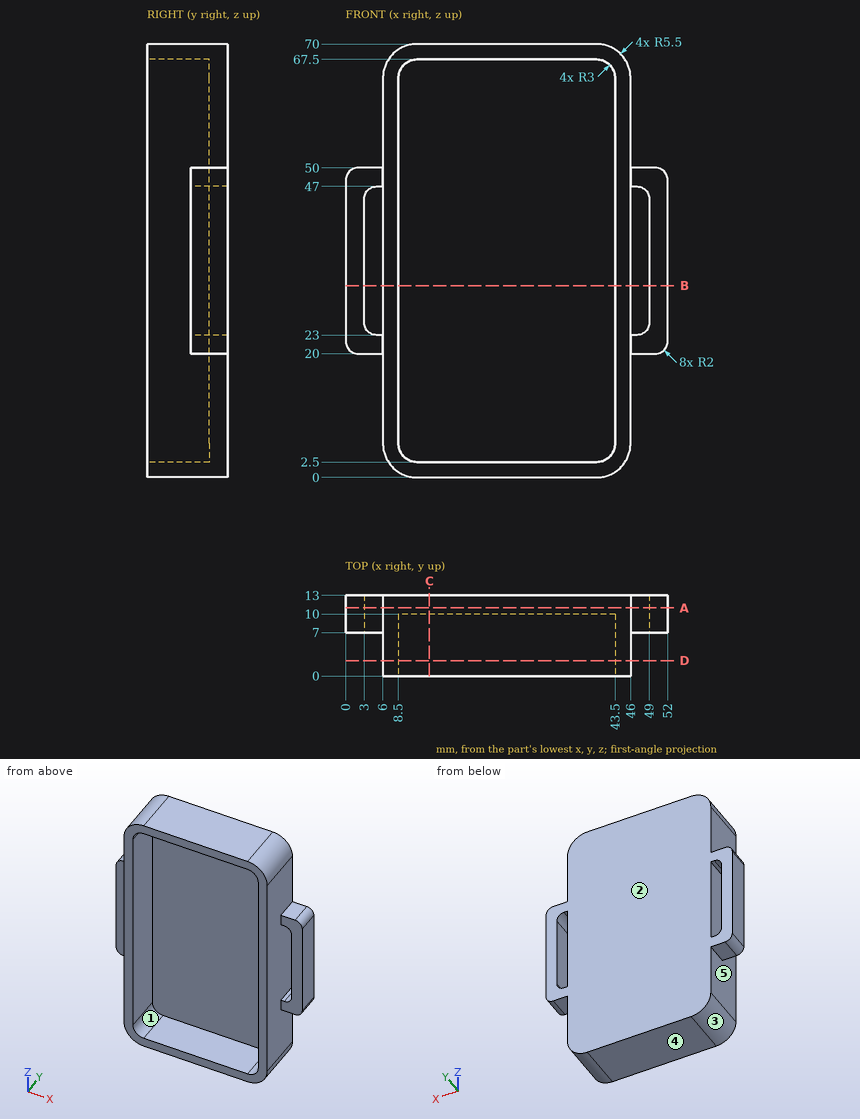
Geometry check sheet. Reference: drawing and pictorial views, mm from the part's lowest x, y, z. A direction names the side the tool comes from. Coordinates: 2 decimals unless noted, no trailing zeros. Order: outer loops, then holes, each group sorted by start corner. A loop starts at its lowest first (then second) coordinate and runs counter-clockwise, first axis right, second up.
1. Sectioned sample at D-D, the plane y = 2.5. Record the cut outline in (x, z), and give its area (3 significant figures).
Results found:
outline: (6, 5.5) arc R5.5 ccw to (11.5, 0) - (40.5, 0) arc R5.5 ccw to (46, 5.5) - (46, 64.5) arc R5.5 ccw to (40.5, 70) - (11.5, 70) arc R5.5 ccw to (6, 64.5) - close; hole (8.5, 5.5) arc R3 ccw to (11.5, 2.5) - (40.5, 2.5) arc R3 ccw to (43.5, 5.5) - (43.5, 64.5) arc R3 ccw to (40.5, 67.5) - (11.5, 67.5) arc R3 ccw to (8.5, 64.5) - close
area: 507 mm2
2. Set-up check for the marked faces 4 and 5: record each of +Z, -Z, +X, -X, +Y, -Y from which the full face is reachable in a straight line by a thin tool's end or side.
Results found:
face 4: -Z, +X, -X, +Y, -Y
face 5: -Y
3. Sectioned sample at B-B, the plane z = 31. Record the cut outline in (x, y), and give its area (3 significant figures).
Results found:
outline: (0, 7) - (3, 7) - (3, 13) - (0, 13) - close; (6, 0) - (8.5, 0) - (8.5, 10) - (43.5, 10) - (43.5, 0) - (46, 0) - (46, 13) - (6, 13) - close; (49, 7) - (52, 7) - (52, 13) - (49, 13) - close
area: 206 mm2
4. Go/stop test with flat-tipped pins: pin 1 Ø1.2 at (x, y) = (4.5, 10) entering from +Z; pin 2 Ø3 at (y, z) = (4.5, 9) entering from -X; pin 3 Ø4.5 at (x, y) = (47, 11) entering from +Z. Record where each tip stops, or that it passes through.
Results found:
pin 1: stops at z = 50
pin 2: stops at x = 6
pin 3: stops at z = 67.99
5. Sectioned sample at A-A, the plane y = 11. Give the number of separate pieces and of enclosed holes in the cut face, and give its area (3 significant figures).
Results found:
separate pieces: 1
enclosed holes: 2
area: 2,990 mm2
6. Release check for a two-part mould opening along Z. For the marked faces 1, 2 and 3 record: +Z half, -Z half, draft (parallel to the pull), parting line (faces both ways), or undercut.
Results found:
face 1: undercut
face 2: draft
face 3: -Z half
7. Sectioned sample at C-C, the plane x = 13.5. Record the cut outline in (y, z), and give its area (3 significant figures).
Results found:
outline: (0, 0) - (13, 0) - (13, 70) - (0, 70) - (0, 67.5) - (10, 67.5) - (10, 2.5) - (0, 2.5) - close
area: 260 mm2
8. Scan lines: line 1 (X direction, y = 10.75, z = 38.5); line 2 (Z direction, x = 30, y = 8.5); line 3 (X direction, y = 6.5, z = 36). Record each from-to range of solid material in increasing order.
Results found:
line 1: x = 0 to 3, 6 to 46, 49 to 52
line 2: z = 0 to 2.5, 67.5 to 70
line 3: x = 6 to 8.5, 43.5 to 46
